The listing builds one solid part. Answer for the finished solid, in the listing's coordinates (mm). Face numbers are marked on the shaded views. A direction names the side the tool comes from. Round coordinates to 2 decimals unless told otherwise and drop trailing zeros. Order: outer loops, then holes, each group sorted by start corner. A loop starts at its lowest first (then second) coordinate and runs counter-clockwise, first axis right, second up. Notation, with made-up numbers: (74, -16) - (96, -16) arc R24 cw to (96, 13) - close; hole circle Ø8 at (1.25, 76). An arc over 180 degrees is marked (long way). Use CSV: the item, a comma, the result in double quotes. Start each with the question number.
Item 1: Find section C-C, the plane y = 30.5. Give the vertices of the cut face in (x, z), plus the area to 3 significant figures.
Item 2: Find section B-B, the plane x = 75. Give the vertices of the cut face in (y, z).
Item 3: Straight lines are drawn through the part: line 1 along X through (y, z) = (183, 46.5); line 2 along Y through (x, z) = (40, 80); line 3 along Z through (x, y) = (97, 131.5). For each, find the intervals that lie inside material, in ascending order. Write a range as [from, to].
Item 4: Find section A-A, the plane z = -1. Give the vertices of the cut face in (x, y), plus the area to 3 significant figures.
Item 5: Flat-ended cylindrical pins translate along their axes: P1, Ø2, axis at x = 115, z = 54.5, coming from the +Y side; P2, Ø7.5, axis at y = 199, z = 75.5, coming from the -X side; P3, Ø3, axis at x = 68.5, z = -6, coming from the +Y side; P4, Ø10, axis at y = 120, z = 63.5, coming from the -X side. Find the tip coordinate at first contact, or state that the pin passes through.
Item 6: For the marked faces 4, 5 and 6, determine the directions among +Z, -Z, +X, -X, +Y, -Y from which every point of the face is accessible in a straight line to the end or side of a thin tool.
Item 7: Find section D-D, the plane x = 130. Give the vertices of the cut face in (y, z).
Item 8: Determine the mould class of the marked faces 1, 2 and 3 for opening direction X: +X half, -X half, draft (parallel to the pull), parting line (faces both ways), or undercut.
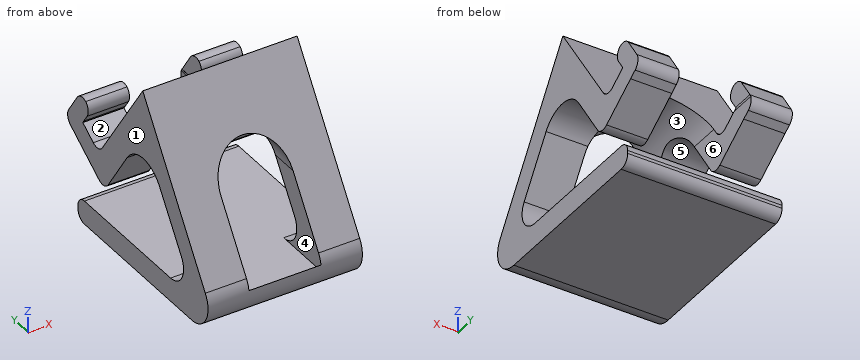
Autodesk Fusion 360 part; units mm, degrees
sketch "Sketch1" plane through (0, 0, 0) normal (1, 0, 0) x (0, 1, 0)
  line L0 (0, 0) -> (100.1869, 151.4759)
  line L1 (100.1869, 151.4759) -> (162.5488, 58.7385)
  line L2 (40.0071, 20.0106) -> (74.3816, 71.287)
  line L3 (124.2987, 71.1676) -> (153.6381, 26.9463)
  line L4 (167.4995, 24.1421) -> (204.4823, 48.679)
  line L5 (176.3756, 55.986) -> (192.5254, 66.7009)
  line L6 (191, 69) -> (192.5254, 66.7009)
  line L7 (0, 0) -> (3.8301, 5.7909)
  line L8 (24.6819, -33.0005) -> (190, -33.0005)
  line L9 (200, -23.0005) -> (200, -20)
  line L10 (190, -10) -> (57.3703, -10)
  line L11 (40.7293, 21.094) -> (39.9929, 19.9893)
  line L12 (191, 69) -> (185.8385, 76.7796)
  line L13 (204.4823, 48.679) -> (211.4637, 53.311)
  line L14 (214.268, 67.1723) -> (201.1527, 86.9401)
  line L15 (188.6427, 90.641) -> (187.2913, 89.7444)
  arc A0 (40.0071, 20.0106) -> (39.9929, 19.9893) centre (48.3134, 14.4423) ccw
  arc A1 (40.7293, 21.094) -> (57.3703, -10) centre (57.3703, 10) ccw
  arc A2 (3.8301, 5.7909) -> (24.6819, -33.0005) centre (24.6819, -8.0005) ccw
  arc A3 (200, -20) -> (190, -10) centre (190, -20) ccw
  arc A4 (190, -33.0005) -> (200, -23.0005) centre (190, -23.0005) ccw
  arc A5 (124.2987, 71.1676) -> (74.3816, 71.287) centre (99.3004, 54.582) ccw
  arc A6 (153.6381, 26.9463) -> (167.4995, 24.1421) centre (161.9709, 32.4749) ccw
  arc A7 (211.4637, 53.311) -> (214.268, 67.1723) centre (205.9352, 61.6438) ccw
  arc A8 (188.6427, 90.641) -> (185.8385, 76.7796) centre (194.1712, 82.3082) ccw
  arc A9 (201.1527, 86.9401) -> (187.2913, 89.7444) centre (192.8199, 81.4116) ccw
  arc A10 (162.5488, 58.7385) -> (176.3756, 55.986) centre (170.8471, 64.3188) ccw
  dimension "d1" = 67.4
  dimension "d2" = 67.4
  dimension "d3" = 10
  dimension "d4" = 20
  dimension "d5" = 25
  dimension "d6" = 10
  dimension "d7" = 30
  dimension "d8" = 10
  dimension "d9" = 10
  dimension "d10" = 10
  dimension "d11" = 10
extrude "Extrude1" add sketch "Sketch1" along normal blind 150 contours L2 L11 A1 | L0 L1 L2 L3 L4 L5 L6 L8 L9 L10 L12 L13 L14 A1 A2 A3 A4 A5 A6 A7 A8 A9 A10
sketch "Sketch2" plane through (0, 0, 0) normal (0, 1, 0) x (1, 0, 0)
  line L0 (110, 10) -> (40, 10)
  line L1 (40, 10) -> (40, -65)
  line L2 (75, -100) -> (75, -100)
  line L3 (110, -65) -> (110, 10)
  arc A0 (40, -65) -> (75, -100) centre (75, -65) ccw
  arc A1 (75, -100) -> (110, -65) centre (75, -65) ccw
  dimension "d14" = 35
extrude "Extrude2" cut sketch "Sketch2" along normal blind 220
ref_plane "WorkPlane1" through (0, 230, 0) normal (0, 1, 0) x (0, 0, 1)
sketch "Sketch3" plane through (0, 230, 0) normal (0, 1, 0) x (1, 0, 0)
  line L0 (40.0833, -92.7367) -> (110.0244, -92.7367)
  line L1 (110.0244, -92.7367) -> (110.0244, -67.17)
  line L2 (110.0244, -67.17) -> (40.0833, -67.17)
  line L3 (40.0833, -67.17) -> (40.0833, -92.7367)
extrude "Extrude3" cut sketch "Sketch3" against normal blind 60
Worked out:
1,outline,"(0, -33) - (150, -33) - (150, 46.11) - (110, 46.11) - (110, -10) - (40, -10) - (40, 46.11) - (0, 46.11) - close"
1,area,"7,940 mm²"
2,outline,"(0, -10) - (0, -4.03) arc R25 ccw to (24.68, -33) - (190, -33) arc R10 ccw to (200, -23) - (200, -20) arc R10 ccw to (190, -10) - close; (66.14, 100) - (134.8, 100) - (100.19, 151.48) - close"
3,line 1,"x = [0, 40], [110, 150]"
3,line 2,"y = [52.91, 83.37], [115.24, 148.25], [184.44, 205.76]"
3,line 3,"z = [-33, -10], [92.22, 104.91]"
4,outline,"(0, 0.68) - (40, 0.68) - (40, 40.67) - (0, 40.67) - close; (110, 0.68) - (150, 0.68) - (150, 40.67) - (110, 40.67) - close"
4,area,"3,200 mm²"
5,P1,"stops at y = 213.83"
5,P2,"stops at x = 0"
5,P3,"stops at y = 0"
5,P4,"passes through"
6,face 4,"+Y"
6,face 5,"+X, -X"
6,face 6,"+Y, -Y"
7,outline,"(3.83, 5.79) arc R25 ccw to (24.68, -33) - (190, -33) arc R10 ccw to (200, -23) - (200, -20) arc R10 ccw to (190, -10) - (57.37, -10) arc R20 cw to (40.55, 20.83) - (74.38, 71.29) arc R30 cw to (124.3, 71.17) - (153.64, 26.95) arc R10 ccw to (167.5, 24.14) - (204.48, 48.68) - (211.46, 53.31) arc R10 ccw to (214.27, 67.17) - (201.15, 86.94) arc R10 ccw to (187.99, 90.17) arc R10 ccw to (185.84, 76.78) - (191, 69) - (192.53, 66.7) - (176.38, 55.99) arc R10 cw to (162.55, 58.74) - (100.19, 151.48) - close"
8,face 1,"-X half"
8,face 2,"draft"
8,face 3,"undercut"
